from build123d import *

# Parameters (mm, degrees)
CYLINDER024_R     = 0.5
CYLINDER024_DEPTH = 20
CYLINDER025_R     = 0.5
CYLINDER025_DEPTH = 20
CYLINDER007_R     = 5
CYLINDER007_DEPTH = 13
PAD006_DEPTH      = 7
SKETCH064_W       = 2
SKETCH064_H       = 3
POCKET006_DEPTH   = 3


with BuildPart() as cylinder024:
    # Cylinder024 → Cylinder024 (new body)
    with BuildSketch(Plane(origin=(39, 12, 17.5), x_dir=(1, 0, 0), z_dir=(0, -1, 0))):
        Circle(CYLINDER024_R)
    extrude(amount=CYLINDER024_DEPTH)


with BuildPart() as fusion025:
    # Cylinder025 → Cylinder025 (new body)
    with BuildSketch(Plane(origin=(49, 12, 17.5), x_dir=(1, 0, 0), z_dir=(0, -1, 0))):
        Circle(CYLINDER025_R)
    extrude(amount=CYLINDER025_DEPTH)

    # Fusion025: union Cylinder024
    add(cylinder024.part)


with BuildPart() as cylinder007:
    # Cylinder007 → Cylinder007 (new body)
    with BuildSketch(Plane(origin=(56, -3, 21), x_dir=(1, 0, 0), z_dir=(0, 1, 0))):
        Circle(CYLINDER007_R)
    extrude(amount=CYLINDER007_DEPTH)


with BuildPart() as potbottommount:
    # Sketch054 → Pad006 (new body)
    with BuildSketch(Plane.XY):
        with BuildLine():
            ThreePointArc((41.408643, 2.758552), (43.911108, 0.256087), (46.413573, 2.758552))
            Line((52.911107, 2.758552), (46.413573, 2.758552))
            Line((52.911107, -3), (52.911107, 2.758552))
            Line((34.911109, -3), (52.911107, -3))
            Line((34.911109, 2.758552), (34.911109, -3))
            Line((41.408643, 2.758552), (34.911109, 2.758552))
        make_face()
    extrude(amount=PAD006_DEPTH)

    # Sketch064 → Pocket006 (cut)
    with BuildSketch(Plane.XY):
        with Locations((35.911109, 2.762661)):
            Rectangle(SKETCH064_W, SKETCH064_H)
    extrude(amount=POCKET006_DEPTH, mode=Mode.SUBTRACT)


with BuildPart() as potbottommount_1:
    # Body006 placement: moved
    add(potbottommount.part.moved(Location((0, 0, 14))))

    # Cut004: cut Cylinder007
    add(cylinder007.part, mode=Mode.SUBTRACT)

    # Cut018: cut Fusion025
    add(fusion025.part, mode=Mode.SUBTRACT)


solid = potbottommount_1.part
Check sheet for the modelled part. Datum: model origin and axes. Units: mm. A direction names the side the tool comes from. Round coordinates to 2 decimals unless told otherwise and drop trailing zeros. Loops run counter-clockwise (first coordinate to the right, second up) from the corner with the lowest first, then second, coordinate; pieces in that order, holes last. Notation, with made-up numbers: (51, -13) -> (71, -13) arc R22 ccw to (71, -3) -> close; hole circle Ø10 at (20, 51). An arc over 180 degrees is marked (long way). Put each result on its own line as item: value. Start each with the question number.
1. Access from +Z, -Z, +X, -X, +Y, -Y to the whole of each face (thin tool, end or side, straight path). Record for faces 5 (the face through (36, 2, 17)), 6 (the face through (39, 0, 18)).
2. Section check A-A (y = -1.15). Enter the section's corners in (x, z).
3. Draft check along X on faces 1 (the face through (36.911, 2, 15)), 2 (the face through (51.517, -0.161, 18.786)), 3 (the face through (43.856, 0.257, 17.451)), 4 (the face through (36, 1.263, 15)). Enter one of: +X half, -X half, draft (parallel to the pull), parting line (faces both ways), or undercut.
4. Section check C-C (z = 17.5). Enter the section's corners in (x, y), plus the area to 3 significant figures.
5. Gauge pin test, flat ends, axial feed: pin 1 (0.7 mm diameter, centred on x = 36, y = 2, fed in from -Z); pin 2 (1 mm diameter, centred on x = 42.5, z = 15.5, fed in from +Y); pin 3 (1.6 mm diameter, centred on x = 36, z = 16, fed in from +Y). Record the tip position at first contact, or that the pin passes through.
6. Section check B-B (x = 49). Enter the section's corners in (y, z).
7. Scan lines: probe 1 along Z at (x, y) = (39, 0.75); probe 2 along X at (y, z) = (0.15, 17.5); probe 3 along X at (y, z) = (1.35, 16.5). Record each from-to range of solid material in increasing order.
8. Section check D-D (y = 0.85). Enter the section's corners in (x, z), plus the area to 3 significant figures.
Findings:
1. face 5: -Z, -X, +Y
1. face 6: +Y, -Y
2. outline: (34.91, 14) -> (52.91, 14) -> (52.91, 17.07) arc R5 cw to (51, 21) -> (34.91, 21) -> close; hole circle Ø1 at (39, 17.5); hole circle Ø1 at (49, 17.5)
3. face 1: -X half
3. face 2: +X half
3. face 3: undercut
3. face 4: draft
4. outline: (34.91, -3) -> (38.5, -3) -> (38.5, 2.76) -> (34.91, 2.76) -> close; (39.5, -3) -> (48.5, -3) -> (48.5, 2.76) -> (46.41, 2.76) arc R2.5 cw to (41.41, 2.76) -> (39.5, 2.76) -> close; (49.5, -3) -> (52.43, -3) -> (52.43, 2.76) -> (49.5, 2.76) -> close
4. area: 79.5 mm^2
5. pin 1: stops at z = 17
5. pin 2: stops at y = 1.14
5. pin 3: stops at y = 1.26
6. outline: (-3, 14) -> (2.76, 14) -> (2.76, 17) -> (-3, 17) -> close; (-3, 18) -> (2.76, 18) -> (2.76, 21) -> (-3, 21) -> close
7. probe 1: z = 14 to 17, 18 to 21
7. probe 2: x = 34.91 to 38.5, 39.5 to 48.5, 49.5 to 52.43
7. probe 3: x = 36.91 to 41.84, 45.98 to 52.91
8. outline: (34.91, 14) -> (42.29, 14) -> (42.29, 21) -> (34.91, 21) -> close; (45.53, 14) -> (52.91, 14) -> (52.91, 17.07) arc R5 cw to (51, 21) -> (45.53, 21) -> close; hole circle Ø1 at (39, 17.5); hole circle Ø1 at (49, 17.5)
8. area: 96.5 mm^2
